Geometry: final body of the model. Coordinates: model frame, mm. Give positions to 0.01 mm unless a question says otherwise; leave off trailing zeros. Order: outer loops, then holes, each group sorted by start corner. A loop starts at its lowest first (then second) coordinate and runs counter-clockwise, first axis right, second up. Notation, with made-up numbers: (40.25, -12.75) - (65.25, -12.75) arc R9 ccw to (65.25, -3.75) - close; hole circle Ø5 at (27.25, -9.5). An arc over 180 degrees is marked (long way). Put each result on its own line as item: value. Start each with the question number.
1. Section D-D on x = -30. Return the cut outline in (y, z).
2. Section C-C on z = -40. Return the cut outline in (x, y), plus the area to 3 significant figures.
3. Section B-B on z = 0. Return the cut outline in (x, y), plus the area to 3 significant figures.
4. Section A-A on x = 0. Return the cut outline in (y, z).
5. Mould query, pull axis X, two halves, no side actions, for faces 1 (the cylindrical face through (15.761, 2.712, 27.445)), 2 (the cylindrical face through (-12.465, 2.712, 56.133)), 3 (the flat face through (12, 5.5, 12)). Classes: pulls with the +X half, pulls with the -X half, needs draft (parallel to the pull), parting line crosses it, or undercut.
6. Ray query, line 1 along Z through (x, y) = (0, 1.25); line 2 along X through (y, z) = (1.8, 20); line 3 along X through (y, z) = (4.55, -25). Return the intervals inside material, ascending. Write a range as from..to.
7. First-contact query: P1, Ø2, axis at y = 4.5, z = -45, coming from the -X side; P2, Ø3, axis at x = 22.5, y = 1, coming from the -Z side. Flat tips, straight axial feed; report the tip coordinate or a pass-through.
from build123d import *

# Parameters (mm, degrees)
SKETCH1_R           = 57.5
SKETCH1_R_2         = 1.65
SKETCH1_R_3         = 2.15
SKETCH1_R_4         = 15
BOSS_EXTRUDE1_DEPTH = 5.5
CHAMFER2_SIZE       = 0.3
SKETCH3_R           = 3.25
CUT_EXTRUDE2_DEPTH  = 10


with BuildPart() as part:
    # Sketch1 → Boss-Extrude1 (new body)
    with BuildSketch(Plane(origin=(0, 0, 0), x_dir=(1, 0, 0), z_dir=(0, 1, 0))):
        Circle(SKETCH1_R)
        with Locations((-30, 0)):
            Circle(SKETCH1_R_2, mode=Mode.SUBTRACT)
        with Locations((-15, 25.980762114)):
            Circle(SKETCH1_R_2, mode=Mode.SUBTRACT)
        with Locations((15, 25.980762114)):
            Circle(SKETCH1_R_2, mode=Mode.SUBTRACT)
        with Locations((30, 0)):
            Circle(SKETCH1_R_2, mode=Mode.SUBTRACT)
        with Locations((15, -25.980762114)):
            Circle(SKETCH1_R_2, mode=Mode.SUBTRACT)
        with Locations((-15, -25.980762114)):
            Circle(SKETCH1_R_2, mode=Mode.SUBTRACT)
        with Locations((-34.641016151, 20)):
            Circle(SKETCH1_R_3, mode=Mode.SUBTRACT)
        with Locations((0, 40)):
            Circle(SKETCH1_R_3, mode=Mode.SUBTRACT)
        with Locations((34.641016151, 20)):
            Circle(SKETCH1_R_3, mode=Mode.SUBTRACT)
        with Locations((34.641016151, -20)):
            Circle(SKETCH1_R_3, mode=Mode.SUBTRACT)
        with Locations((0, -40)):
            Circle(SKETCH1_R_3, mode=Mode.SUBTRACT)
        with Locations((-34.641016151, -20)):
            Circle(SKETCH1_R_3, mode=Mode.SUBTRACT)
        Circle(SKETCH1_R_4, mode=Mode.SUBTRACT)
    extrude(amount=BOSS_EXTRUDE1_DEPTH)

    # Chamfer2
    chamfer2_edges = [part.edges().sort_by_distance(p)[0] for p in [
        (-15, 0, 0),
        (-15, 5.5, 0),
    ]]
    chamfer(chamfer2_edges, length=CHAMFER2_SIZE)

    # Sketch3 → Cut-Extrude2 (cut)
    with BuildSketch(Plane.XZ):
        with Locations((24.248711306, -14)):
            Circle(SKETCH3_R)
    extrude(amount=-CUT_EXTRUDE2_DEPTH, mode=Mode.SUBTRACT)


solid = part.part
Resolved:
1. outline: (0, -49.05) - (5.5, -49.05) - (5.5, -1.65) - (0, -1.65) - close; (0, 1.65) - (5.5, 1.65) - (5.5, 49.05) - (0, 49.05) - close
2. outline: (-41.31, 0) - (-2.15, 0) - (-2.15, 5.5) - (-41.31, 5.5) - close; (2.15, 0) - (41.31, 0) - (41.31, 5.5) - (2.15, 5.5) - close
2. area: 431 mm^2
3. outline: (-57.5, 0) - (-31.65, 0) - (-31.65, 5.5) - (-57.5, 5.5) - close; (-28.35, 0) - (-15.3, 0) - (-15, 0.3) - (-15, 5.2) - (-15.3, 5.5) - (-28.35, 5.5) - close; (15, 0.3) - (15.3, 0) - (28.35, 0) - (28.35, 5.5) - (15.3, 5.5) - (15, 5.2) - close; (31.65, 0) - (57.5, 0) - (57.5, 5.5) - (31.65, 5.5) - close
3. area: 431 mm^2
4. outline: (0, -57.5) - (5.5, -57.5) - (5.5, -42.15) - (0, -42.15) - close; (0, -37.85) - (5.5, -37.85) - (5.5, -15.3) - (5.2, -15) - (0.3, -15) - (0, -15.3) - close; (0, 15.3) - (0.3, 15) - (5.2, 15) - (5.5, 15.3) - (5.5, 37.85) - (0, 37.85) - close; (0, 42.15) - (5.5, 42.15) - (5.5, 57.5) - (0, 57.5) - close
5. face 1: undercut
5. face 2: parting line crosses it
5. face 3: needs draft
6. line 1: -57.5..-42.15, -37.85..-15, 15..37.85, 42.15..57.5
6. line 2: -53.91..-36.79, -32.49..32.49, 36.79..53.91
6. line 3: -51.78..-16.33, -13.67..13.67, 16.33..51.78
7. P1: x = -37.02
7. P2: z = -53.53
